from build123d import *

# Parameters (mm, degrees)
SKETCH_1_R            = 55
EXTRUDE_1_DEPTH       = 5
SKETCH_2_R            = 49.9
EXTRUDE_2_DEPTH       = 3
SKETCH_3_W            = 35
SKETCH_3_H            = 30
EXTRUDE_3_DEPTH       = 25
SKETCH_5_R            = 4.1
CUT_EXTRUDE_2_DEPTH   = 9
SKETCH_6_R            = 2.75
CUT_EXTRUDE_3_DEPTH   = 34
SKETCH2_W             = 20.25
SKETCH2_H             = 10.35
CUT_EXTRUDE1_DEPTH    = 73.5
SKETCH3_W             = 17.5
SKETCH3_H             = 27.9
SKETCH3_W_2           = 48.3
SKETCH3_H_2           = 25.3
CUT_EXTRUDE2_DEPTH    = 4
CHAMFER1_SIZE         = 2
CHAMFER1_SIZE2        = 0.535898385
CHAMFER1_PART_2_SIZE  = 2
CHAMFER1_PART_2_SIZE2 = 0.535898385
CHAMFER1_PART_3_SIZE  = 2
CHAMFER1_PART_3_SIZE2 = 0.535898385
CHAMFER1_PART_4_SIZE  = 2
CHAMFER1_PART_4_SIZE2 = 0.535898385
SKETCH4_W             = 35
SKETCH4_H             = 30
CUT_EXTRUDE3_DEPTH    = 12.5
BOSS_EXTRUDE2_START   = -2
SKETCH5_W             = 20
SKETCH5_H             = 70
BOSS_EXTRUDE2_DEPTH   = 5.325
SKETCH6_R             = 4.15
CUT_EXTRUDE4_DEPTH    = 14.3250001
CUT_EXTRUDE5_DEPTH    = 6.5
CHAMFER2_SIZE         = 1
CHAMFER2_SIZE2        = 2.747477419
SKETCH8_R             = 1.5
CUT_EXTRUDE6_DEPTH    = 17.5


with BuildPart() as part:
    # Эскиз1 → Бобышка-Вытянуть1 (new body)
    with BuildSketch(Plane(origin=(0, 0, 0), x_dir=(1, 0, 0), z_dir=(0, 1, 0))):
        with Locations(Location((0, 0, 0), (0, 0, 270))):  # turned: the seam where the file's is
            Circle(SKETCH_1_R)
    extrude(amount=EXTRUDE_1_DEPTH)

    # Эскиз2 → Бобышка-Вытянуть2 (add)
    with BuildSketch(Plane(origin=(0, 5, 0), x_dir=(1, 0, 0), z_dir=(0, 1, 0))):
        with Locations(Location((0, 0, 0), (0, 0, 270))):  # turned: the seam where the file's is
            Circle(SKETCH_2_R)
    extrude(amount=EXTRUDE_2_DEPTH)

    # Эскиз3 → Бобышка-Вытянуть3 (add)
    with BuildSketch(Plane.XZ):
        Rectangle(SKETCH_3_W, SKETCH_3_H)
    extrude(amount=EXTRUDE_3_DEPTH)

    # Эскиз5 → Вырез-Вытянуть2 (cut, through all)
    with BuildSketch(Plane.XZ):
        with Locations(Location((33.592198598, -32.871936263, 0), (0, 0, 270))):  # turned: the seam where the file's is
            Circle(SKETCH_5_R)
        with Locations(Location((-33.591727056, -32.872418125, 0), (0, 0, 270))):  # turned: the seam where the file's is
            Circle(SKETCH_5_R)
        with Locations(Location((-33.591727056, 32.872418125, 0), (0, 0, 270))):  # turned: the seam where the file's is
            Circle(SKETCH_5_R)
        with Locations(Location((33.483215177, 32.983215177, 0), (0, 0, 270))):  # turned: the seam where the file's is
            Circle(SKETCH_5_R)
    extrude(amount=-CUT_EXTRUDE_2_DEPTH, mode=Mode.SUBTRACT)

    # Эскиз6 → Вырез-Вытянуть3 (cut, through all)
    with BuildSketch(Plane(origin=(0, 8, 0), x_dir=(1, 0, 0), z_dir=(0, 1, 0))):
        with Locations(Location((-17.999856554, 19.999999999, 0), (0, 0, 270))):  # turned: the seam where the file's is
            Circle(SKETCH_6_R)
    extrude(amount=-CUT_EXTRUDE_3_DEPTH, mode=Mode.SUBTRACT)

    # Sketch2 → Cut-Extrude1 (cut, through all)
    with BuildSketch(Plane.ZY.offset(17.5)):
        with Locations((0, -12.5)):
            Rectangle(SKETCH2_W, SKETCH2_H)
    extrude(amount=-CUT_EXTRUDE1_DEPTH, mode=Mode.SUBTRACT)

    # Sketch3 → Cut-Extrude2 (cut)
    with BuildSketch(Plane(origin=(0, 8, 0), x_dir=(1, 0, 0), z_dir=(0, 1, 0))):
        with Locations((35, 0)):
            Rectangle(SKETCH3_W, SKETCH3_H)
        Rectangle(SKETCH3_W_2, SKETCH3_H_2)
    extrude(amount=-CUT_EXTRUDE2_DEPTH, mode=Mode.SUBTRACT)

    # Chamfer1
    chamfer1_edges = [part.edges().sort_by_distance(p)[0] for p in [
        (0.000357897, 8, -49.899999999),
    ]]
    chamfer1_side = [part.faces().sort_by_distance(p)[0] for p in [
        (0.000357897, 6.5, -49.899999999),
    ]]
    chamfer(chamfer1_edges, length=CHAMFER1_SIZE, length2=CHAMFER1_SIZE2, reference=chamfer1_side[0])

    # Chamfer1 part 2
    chamfer1_part_2_edges = [part.edges().sort_by_distance(p)[0] for p in [
        (-49.9, 8, 0),
    ]]
    chamfer1_part_2_side = [part.faces().sort_by_distance(p)[0] for p in [
        (-49.9, 6.5, 0),
    ]]
    chamfer(chamfer1_part_2_edges, length=CHAMFER1_PART_2_SIZE, length2=CHAMFER1_PART_2_SIZE2, reference=chamfer1_part_2_side[0])

    # Chamfer1 part 3
    chamfer1_part_3_edges = [part.edges().sort_by_distance(p)[0] for p in [
        (-0.08242255, 8, 49.899931929),
    ]]
    chamfer1_part_3_side = [part.faces().sort_by_distance(p)[0] for p in [
        (-0.08242255, 6.5, 49.899931929),
    ]]
    chamfer(chamfer1_part_3_edges, length=CHAMFER1_PART_3_SIZE, length2=CHAMFER1_PART_3_SIZE2, reference=chamfer1_part_3_side[0])

    # Chamfer1 part 4
    chamfer1_part_4_edges = [part.edges().sort_by_distance(p)[0] for p in [
        (49.899931657, 8, 0.082587101),
    ]]
    chamfer1_part_4_side = [part.faces().sort_by_distance(p)[0] for p in [
        (49.899931657, 6.5, 0.082587101),
    ]]
    chamfer(chamfer1_part_4_edges, length=CHAMFER1_PART_4_SIZE, length2=CHAMFER1_PART_4_SIZE2, reference=chamfer1_part_4_side[0])

    # Sketch4 → Cut-Extrude3 (cut)
    with BuildSketch(Plane.XZ.offset(25)):
        Rectangle(SKETCH4_W, SKETCH4_H)
    extrude(amount=-CUT_EXTRUDE3_DEPTH, mode=Mode.SUBTRACT)

    # Sketch5 → Boss-Extrude2 (add)
    with BuildSketch(Plane.XZ.offset(7.325).offset(BOSS_EXTRUDE2_START)):
        Rectangle(SKETCH5_W, SKETCH5_H)
    extrude(amount=-BOSS_EXTRUDE2_DEPTH)

    # Sketch6 → Cut-Extrude4 (cut, through all)
    with BuildSketch(Plane.XZ.offset(5.325)):
        with Locations(Location((0, 25, 0), (0, 0, 270))):  # turned: the seam where the file's is
            Circle(SKETCH6_R)
        with Locations(Location((0, -25, 0), (0, 0, 270))):  # turned: the seam where the file's is
            Circle(SKETCH6_R)
    extrude(amount=-CUT_EXTRUDE4_DEPTH, mode=Mode.SUBTRACT)

    # Sketch7 → Cut-Extrude5 (cut)
    with BuildSketch(Plane(origin=(0, 8, 0), x_dir=(1, 0, 0), z_dir=(0, 1, 0))):
        Polygon((0, -32.5), (6.495190528, -28.75), (6.495190528, -21.25), (0, -17.5), (-6.495190528, -21.25), (-6.495190528, -28.75), align=None)
        Polygon((0, 17.5), (6.495190528, 21.25), (6.495190528, 28.75), (0, 32.5), (-6.495190528, 28.75), (-6.495190528, 21.25), align=None)
    extrude(amount=-CUT_EXTRUDE5_DEPTH, mode=Mode.SUBTRACT)

    # Chamfer2
    chamfer2_edges = [part.edges().sort_by_distance(p)[0] for p in [
        (-3.247595264, 8, 30.625),
        (3.247595264, 8, 30.625),
        (6.495190528, 8, 25),
        (3.247595264, 8, 19.375),
        (-3.247595264, 8, 19.375),
        (-6.495190528, 8, 25),
        (-3.247595264, 8, -19.375),
        (3.247595264, 8, -19.375),
        (6.495190528, 8, -25),
        (3.247595264, 8, -30.625),
        (-3.247595264, 8, -30.625),
        (-6.495190528, 8, -25),
    ]]
    chamfer2_side = [part.faces().sort_by_distance(p)[0] for p in [
        (36.933184569, 8, 28.704637204),
    ]]
    chamfer(chamfer2_edges, length=CHAMFER2_SIZE, length2=CHAMFER2_SIZE2, reference=chamfer2_side[0])

    # Sketch8 → Cut-Extrude6 (cut, through all)
    with BuildSketch(Plane(origin=(0, 4, 0), x_dir=(1, 0, 0), z_dir=(0, 1, 0))):
        with Locations(Location((20, 9, 0), (0, 0, 270))):  # turned: the seam where the file's is
            Circle(SKETCH8_R)
        with Locations(Location((20, -9, 0), (0, 0, 270))):  # turned: the seam where the file's is
            Circle(SKETCH8_R)
        with Locations(Location((-20, 9, 0), (0, 0, 270))):  # turned: the seam where the file's is
            Circle(SKETCH8_R)
        with Locations(Location((-20, -9, 0), (0, 0, 270))):  # turned: the seam where the file's is
            Circle(SKETCH8_R)
    extrude(amount=-CUT_EXTRUDE6_DEPTH, mode=Mode.SUBTRACT)


solid = part.part
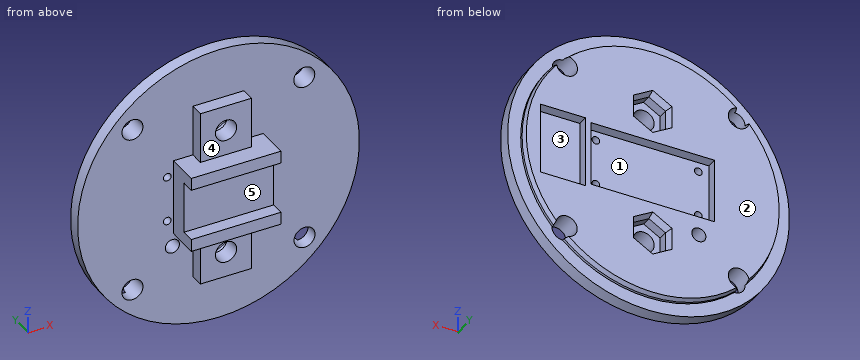
Could you check a few things on this model? Use its own coordinates, in mm. Face numbers are marked on the shaded views. A direction names the side the tool comes from. Round coordinates to 2 decimals unless told otherwise and drop trailing zeros. Use a Markdown table: item, result.
Q1. I want a section at A-A (x = -31.5). Count the separate pieces of the cut face and the enclosed holes in it, plus the area to 3 significant figures.
Output values:
| item | result |
|---|---|
| separate pieces | 3 |
| enclosed holes | 0 |
| area | 569 mm2 |
Q2. Please list where these lines run through material, in increasing order: L1, parallel to X at y = 2.15, z = 9; L2, parallel to X at y = -0.5, z = 25; L3, parallel to X at y = 1.5, z = 34.5.
Output values:
| item | result |
|---|---|
| L1 | -54.26 to -21.5, -18.5 to 18.5, 21.5 to 54.26 |
| L2 | -10 to -4.15, 4.15 to 10 |
| L3 | -42.83 to -37.35, -29.83 to 29.67, 37.29 to 42.83 |
Q3. For the marked faces 3, 4 and 5, which set-ups out of +Z, -Z, +X, -X, +Y, -Y let a thin tool reach every point of the face, with its end or its side?
Output values:
| item | result |
|---|---|
| face 3 | +Y |
| face 4 | +Z, +X, -X, -Y |
| face 5 | +X, -X, -Y |
Q4. For pin 1 (1.8 mm diameter, centred on x = 20, z = -9, fed in from +Y); pin 2 (16 mm diameter, centred on x = 4, z = 2, fed in from -Y) (3 decimals); pin 3 (1.2 mm diameter, centred on x = 34, y = 7, fed in from +Z); pin 4 (12 mm diameter, centred on x = -2, z = -26, fed in from -Y) (3 decimals), each with a flat end and sliding along its axis, tell me the tip position at first contact or that it passes through.
Output values:
| item | result |
|---|---|
| pin 1 | through |
| pin 2 | y = -7.325 |
| pin 3 | z = 29.04 |
| pin 4 | y = -5.325 |
Q5. Thinking about a two-plate mould opening in X: for the marked faces 1 and 2, which applies, released by +X, released by -X, zero draft, split by the parting line, or undercut?
Output values:
| item | result |
|---|---|
| face 1 | undercut |
| face 2 | zero draft |
